Geometry: final body of the model. Coordinates: model frame, mm. A direction names the side the tool comes from. Give positions to 0.01 mm unless a question says otherwise; leave off trailing zeros. Write each loop counter-clockwise with the first axis right and the second up, starting at its lowest first coordinate (ties: lowest second). Pieces come first, ordered by that corner, then holes. Notation, with made-up numbers: (-5, 21) -> (40, 21) arc R29 ccw to (40, 53) -> close; hole circle Ø2 at (59, 78.5). An arc over 180 degrees is marked (long way). Answer in a Markdown table with one row per item. Add a question column.
Item 1: Section query C-C on x = 2.5. Output: boundary loops of the cut face in (y, z).
Item 2: Material intervals for probe 1 along X at (y, z) = (-27.5, 5.75); probe 2 along Z at (x, y) = (-3.25, -12); probe 3 along Y at (x, z) = (-7.75, 14), sorted ascending. Write a range as from..to.
Item 3: Section query A-A on z = 11.75. Output: boundary loops of the cut face in (x, y).
Item 4: Section query B-B on y = -7. Output: boundary loops of the cut face in (x, z).
Item 5: Section query D-D on z = 16.5. Output: boundary loops of the cut face in (x, y), plus the area to 3 significant figures.
Item 6: Access query for faces 1 (the flat face through (5, -27, 3)), 2 (the flat face through (0, -18, 11)), 3 (the flat face through (5, -5, 14)). Directions: +Z, -Z, +X, -X, +Y, -Y. A direction counts if a zero-diameter tool reaches every point of the face in a straight line with its end or side. Return the directions, or none.
Item 7: First-contact query: P1, Ø3, axis at x = -0.5, y = -24, coming from the +Z side; P2, Ø1, axis at x = 3, y = -13.5, coming from the +Z side. Flat tips, straight axial feed; report the tip coordinate or a pass-through.
Item 8: Draft query along X for faces 4 (the flat face through (10, -11, 8)), 5 (the flat face through (0, 0, 8)), 6 (the flat face through (-5, -27, 3)), 7 (the flat face through (-0.07, -23.744, 3.669)). Return one class per face: +X half, -X half, draft (parallel to the pull), parting line (faces both ways), or undercut.
```python
from build123d import *

# Parameters (mm, degrees)
F1_DEPTH = 30
F3_DEPTH = 20.001
F5_DEPTH = 5
F6_W     = 10
F6_H     = 5
F7_DEPTH = 17.88954382


with BuildPart() as f1:
    # F0 (on Front) → F1 (new body)
    with BuildSketch(Plane.XZ):
        Polygon((-10, 20), (-10, 0), (10, 0), (10, 20), (5, 20), (5, 11.2048187231), (-5, 11.2048187231), (-5, 20), align=None)
    extrude(amount=F1_DEPTH)

    # F2 (on face) → F3 (cut, through all)
    with BuildSketch(Plane(origin=(-10, 0, 0), x_dir=(0, -1, 0), z_dir=(-1, 0, 0))):
        Polygon((0, 20), (30, 5), (30, 20), align=None)
    extrude(amount=-F3_DEPTH, mode=Mode.SUBTRACT)

    # F4 (on face) → F5 (cut)
    with BuildSketch(Plane.XZ.offset(30)):
        Polygon((-5, 2.5), (-5, 0), (5, 0), (5, 2.5), (5, 5), (-5, 5), align=None)
    extrude(amount=-F5_DEPTH, mode=Mode.SUBTRACT)

    # F6 (on face) → F7 (cut, through all)
    with BuildSketch(Plane(origin=(0, -8, 16), x_dir=(1, 0, 0), z_dir=(0, -0.4472135955, 0.894427191))):
        with Locations((0, -22.0967477525)):
            Rectangle(F6_W, F6_H)
    extrude(amount=-F7_DEPTH, mode=Mode.SUBTRACT)


solid = f1.part
```
Findings below:
| question | item | result |
|---|---|---|
| 1 | outline | (-25.53, 7.24) -> (-21.91, 0) -> (0, 0) -> (0, 11.2) -> (-17.59, 11.2) -> close |
| 2 | probe 1 | x = -10..-5, 5..10 |
| 2 | probe 2 | z = 0..11.2 |
| 2 | probe 3 | y = -12..0 |
| 3 | outline | (-10, -16.5) -> (-5, -16.5) -> (-5, 0) -> (-10, 0) -> close; (5, -16.5) -> (10, -16.5) -> (10, 0) -> (5, 0) -> close |
| 4 | outline | (-10, 0) -> (10, 0) -> (10, 16.5) -> (5, 16.5) -> (5, 11.2) -> (-5, 11.2) -> (-5, 16.5) -> (-10, 16.5) -> close |
| 5 | outline | (-10, -7) -> (-5, -7) -> (-5, 0) -> (-10, 0) -> close; (5, -7) -> (10, -7) -> (10, 0) -> (5, 0) -> close |
| 5 | area | 70.0 mm^2 |
| 6 | face 1 | -Z, -Y |
| 6 | face 2 | +Z, +X, -X, -Y |
| 6 | face 3 | +Z, +Y, -Y |
| 7 | P1 | stops at z = 8.75 |
| 7 | P2 | stops at z = 11.2 |
| 8 | face 4 | +X half |
| 8 | face 5 | draft |
| 8 | face 6 | undercut |
| 8 | face 7 | undercut |
